Could you check a few things on this model? Use its own coordinates, in mm. A direction names the side the tool comes from. Round coordinates to 2 decimals unless told otherwise and drop trailing zeros. Loops run counter-clockwise (first coordinate to the right, second up) from the corner with the lowest first, then second, coordinate; pieces in that order, holes last. Notation, with made-up numbers: (10.25, -16) - (64.25, -16) arc R14 ccw to (64.25, 9) - close; hole circle Ø4 at (42, 16). An arc over 180 degrees is marked (long way). Answer as CSV lines item,"result". Start each with the question number.
1) Suppose I cut it at A-A, the plane z = 35. Write out the boundary of the cut face in (x, y).
2) Suppose I cut it at C-C, the plane x = 15. Write out the boundary of the cut face in (y, z) (3 decimals), then the cut area to 3 significant figures.
3) Which directions (+Z, -Z, +X, -X, +Y, -Y) give clear straight access to the entire face, cutting with the end or side of a thin tool? Please do faces 1 (the face through (0, 0, 27)), 2 (the face through (0, 5.1, 0)).
4) Suppose I cut it at B-B, the plane y = 14.75. Write out the boundary of the cut face in (x, z), then the cut area to 3 significant figures.
5) I'm going to push a flat-ended pin straight in: pin 1 Ø5 at (x, z) = (15, -35) entering from -Y. Where does the tip first touch, or does it pass through?
6) Suppose I cut it at D-D, the plane x = -5. Write out the boundary of the cut face in (y, z) (3 decimals), then the cut area to 3 significant figures.
7) Please list where these lines run through material, in increasing order: line 1 along X through (y, z) = (12, -35); line 2 along X through (y, z) = (4.75, -34); line 3 along Z through (x, y) = (-6, 3.25) (3 decimals).
8) We'd pull the mould along Z, two halves only. Please class faces 3 (the face through (0, 10, -45)), 4 (the face through (25, 10, 1)), 5 (the face through (0, 3, -10.125)): pulls with the +Z half, pulls with the -Z half, needs draft (parallel to the pull), parting line crosses it, or undercut.
```python
from build123d import *
from OCP.BRepFilletAPI import BRepFilletAPI_MakeChamfer

# Parameters (mm, degrees)
SKETCH1_W               = 50
SKETCH1_H               = 90
BOSS_EXTRUDE1_DEPTH     = 20
CUT_EXTRUDE1_DEPTH      = 71.178344238
CUT_EXTRUDE1_DEPTH_BACK = 71.178344238
SKETCH2_W               = 20.25
SKETCH2_H               = 5.1
SKETCH3_R               = 4.15
CUT_EXTRUDE2_DEPTH      = 56.226805086
CHAMFER1_SIZE           = 1
CHAMFER1_SIZE2          = 0.577350269


with BuildPart() as part:
    # Sketch1 → Boss-Extrude1 (new body)
    with BuildSketch(Plane(origin=(0, 0, 0), x_dir=(1, 0, 0), z_dir=(0, 1, 0))):
        Rectangle(SKETCH1_W, SKETCH1_H)
    extrude(amount=BOSS_EXTRUDE1_DEPTH)

    # Sketch2 → Cut-Extrude1 (cut, two sides: drawn at the far end of the back side and taken through both)
    with BuildSketch(Plane(origin=(25, 0, 0), x_dir=(0, 0, -1), z_dir=(1, 0, 0)).offset(-CUT_EXTRUDE1_DEPTH_BACK)):
        with Locations((0, 2.55)):
            Rectangle(SKETCH2_W, SKETCH2_H)
    extrude(amount=CUT_EXTRUDE1_DEPTH + CUT_EXTRUDE1_DEPTH_BACK, mode=Mode.SUBTRACT)

    # Sketch3 → Cut-Extrude2 (cut, through all)
    with BuildSketch(Plane.XZ):
        with Locations(Location((-15, 35, 0), (0, 0, 270))):
            Circle(SKETCH3_R)
        with Locations(Location((-15, -35, 0), (0, 0, 270))):
            Circle(SKETCH3_R)
        with Locations(Location((15, 35, 0), (0, 0, 270))):
            Circle(SKETCH3_R)
        with Locations(Location((15, -35, 0), (0, 0, 270))):
            Circle(SKETCH3_R)
    extrude(amount=-CUT_EXTRUDE2_DEPTH, mode=Mode.SUBTRACT)

    # Chamfer1: one chamfer whose edges measure the first distance from different faces: ONE call of the kernel's chamfer builder (chamfer() names one face for all edges)
    chamfer1_edges_1 = [part.edges().sort_by_distance(p)[0] for p in [
        (-15, 20, 39.15),
    ]]
    chamfer1_side_1 = [part.faces().sort_by_distance(p)[0] for p in [
        (-15, 10, 39.15),
    ]]
    chamfer1_edges_2 = [part.edges().sort_by_distance(p)[0] for p in [
        (15, 20, 39.15),
    ]]
    chamfer1_side_2 = [part.faces().sort_by_distance(p)[0] for p in [
        (15, 10, 39.15),
    ]]
    chamfer1_edges_3 = [part.edges().sort_by_distance(p)[0] for p in [
        (15, 20, -30.85),
    ]]
    chamfer1_side_3 = [part.faces().sort_by_distance(p)[0] for p in [
        (15, 10, -30.85),
    ]]
    chamfer1_edges_4 = [part.edges().sort_by_distance(p)[0] for p in [
        (-15, 20, -30.85),
    ]]
    chamfer1_side_4 = [part.faces().sort_by_distance(p)[0] for p in [
        (-15, 10, -30.85),
    ]]
    chamfer1 = BRepFilletAPI_MakeChamfer(part.part.solid().wrapped)
    for e in chamfer1_edges_1:
        chamfer1.Add(CHAMFER1_SIZE, CHAMFER1_SIZE2, e.wrapped, chamfer1_side_1[0].wrapped)  # the first distance lies on this face
    for e in chamfer1_edges_2:
        chamfer1.Add(CHAMFER1_SIZE, CHAMFER1_SIZE2, e.wrapped, chamfer1_side_2[0].wrapped)  # the first distance lies on this face
    for e in chamfer1_edges_3:
        chamfer1.Add(CHAMFER1_SIZE, CHAMFER1_SIZE2, e.wrapped, chamfer1_side_3[0].wrapped)  # the first distance lies on this face
    for e in chamfer1_edges_4:
        chamfer1.Add(CHAMFER1_SIZE, CHAMFER1_SIZE2, e.wrapped, chamfer1_side_4[0].wrapped)  # the first distance lies on this face
    add(Compound.cast(chamfer1.Shape()), mode=Mode.REPLACE)


solid = part.part
```
Filled sheet:
1,outline,"(-25, 0) - (-19.15, 0) - (-19.15, 19) - (-19.73, 20) - (-25, 20) - close; (-10.85, 0) - (10.85, 0) - (10.85, 19) - (10.27, 20) - (-10.27, 20) - (-10.85, 19) - close; (19.15, 0) - (25, 0) - (25, 20) - (19.73, 20) - (19.15, 19) - close"
2,outline,"(0, -45) - (20, -45) - (20, -39.727) - (19, -39.15) - (0, -39.15) - close; (0, -30.85) - (19, -30.85) - (20, -30.273) - (20, 30.273) - (19, 30.85) - (0, 30.85) - (0, 10.125) - (5.1, 10.125) - (5.1, -10.125) - (0, -10.125) - close; (0, 39.15) - (19, 39.15) - (20, 39.727) - (20, 45) - (0, 45) - close"
2,area,"1,360 mm²"
3,face 1,"+Z, -Z, +X, -X, -Y"
3,face 2,"+X, -X, -Y"
4,outline,"(-25, -45) - (25, -45) - (25, 45) - (-25, 45) - close; hole circle Ø8.3 at (-15, -35); hole circle Ø8.3 at (-15, 35); hole circle Ø8.3 at (15, -35); hole circle Ø8.3 at (15, 35)"
4,area,"4,280 mm²"
5,pin 1,"through"
6,outline,"(0, -45) - (20, -45) - (20, 45) - (0, 45) - (0, 10.125) - (5.1, 10.125) - (5.1, -10.125) - (0, -10.125) - close"
6,area,"1,700 mm²"
7,line 1,"-25 to -19.15, -10.85 to 10.85, 19.15 to 25"
7,line 2,"-25 to -19.03, -10.97 to 10.97, 19.03 to 25"
7,line 3,"-45 to -10.125, 10.125 to 45"
8,face 3,"pulls with the -Z half"
8,face 4,"needs draft"
8,face 5,"undercut"
